Could you check a few things on this drawing? It's one solid part, dimensions in mm from its lowest x, y, z. A direction names the side the tool comes from. Give positions to 0.01 mm unless a question says otherwise; leave off trailing zeros. Order: outer loops, then holes, each group sorted by start corner. A loop starts at its lowest first (then second) coordinate and runs counter-clockwise, first axis right, second up.
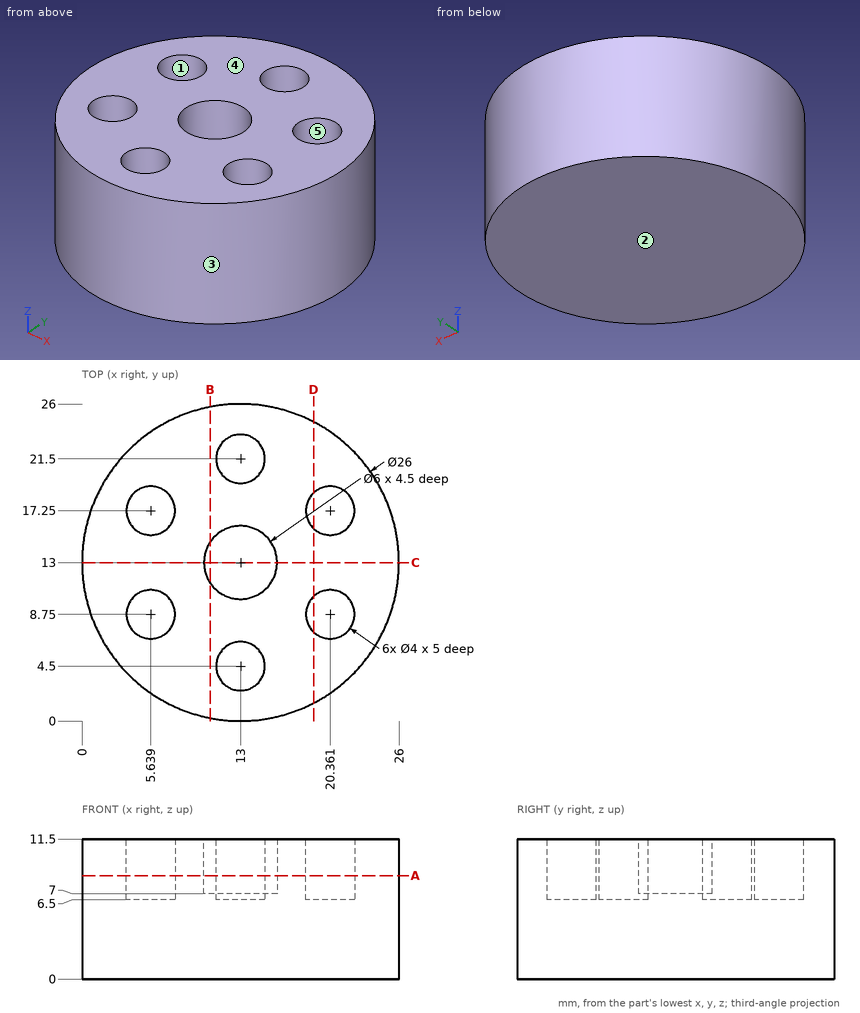
Q1. If we section it at B-B on x = 10.5: List the corners of the cut face in (y, z) for me, plus the area to 4 significant figures.
Filled sheet:
outline: (0.24, 0) - (25.76, 0) - (25.76, 11.5) - (14.66, 11.5) - (14.66, 7) - (11.34, 7) - (11.34, 11.5) - (0.24, 11.5) - close
area: 278.5 mm2
Q2. I need wall thicknesses on L1, parallel to Y at x = 13, z = 10.35; L2, parallel to Y at x = 19, z = 8.5 (1 decimal); L3, parallel to Y at x = 4.25, z = 8 (1 decimal). Which ranges of each line are inside material? Lowest first, please.
Filled sheet:
L1: y = 0 to 2.5, 6.5 to 10, 16 to 19.5, 23.5 to 26
L2: y = 1.5 to 7.3, 10.2 to 15.8, 18.7 to 24.5
L3: y = 3.4 to 7.3, 10.2 to 15.8, 18.7 to 22.6
Q3. If we section it at A-A on z = 8.5: List the corners of the cut face in (x, y) for me.
Filled sheet:
outline: circle Ø26 at (13, 13); hole circle Ø4 at (5.64, 8.75); hole circle Ø4 at (5.64, 17.25); hole circle Ø6 at (13, 13); hole circle Ø4 at (13, 4.5); hole circle Ø4 at (13, 21.5); hole circle Ø4 at (20.36, 8.75); hole circle Ø4 at (20.36, 17.25)
Q4. If we section it at D-D on x = 19: List the corners of the cut face in (y, z) for me (1 decimal).
Filled sheet:
outline: (1.5, 0) - (24.5, 0) - (24.5, 11.5) - (18.7, 11.5) - (18.7, 6.5) - (15.8, 6.5) - (15.8, 11.5) - (10.2, 11.5) - (10.2, 6.5) - (7.3, 6.5) - (7.3, 11.5) - (1.5, 11.5) - close
Q5. For the marked faces 4 and 5, which set-ups out of +Z, -Z, +X, -X, +Y, -Y let a thin tool reach every point of the face, with its end or its side?
Filled sheet:
face 4: +Z, +X, -X, +Y, -Y
face 5: +Z
Q6. If we section it at C-C on y = 13: List the corners of the cut face in (x, z) for me, plus the area to 3 significant figures.
Filled sheet:
outline: (0, 0) - (26, 0) - (26, 11.5) - (16, 11.5) - (16, 7) - (10, 7) - (10, 11.5) - (0, 11.5) - close
area: 272 mm2
Q7. Thinking about a two-plate mould opening in X: for the marked faces 1, 2 and 3, which applies, released by +X, released by -X, zero draft, split by the parting line, or undercut?
Filled sheet:
face 1: undercut
face 2: zero draft
face 3: split by the parting line
Q8. I'm going to push flat-ended pins straight in: P1, Ø6.5, axis at x = 13, y = 4.5, coming from the +Z side; P2, Ø5, axis at y = 19.5, z = 9, coming from the -X side; P3, Ø1.5, axis at x = 6, z = 7, coming from the -Y side; P4, Ø4, axis at y = 8, z = 1.5, coming from the +X side. Where does each tip first touch, or does it pass through?
Filled sheet:
P1: stops at z = 11.5
P2: stops at x = 0.63
P3: stops at y = 1.6
P4: stops at x = 25.65
